Geometry check sheet. Reference: drawing and pictorial views, mm from the part's lowest x, y, z. A direction names the side the tool comes from. Coordinates: 2 decimals unless noted, no trailing zeros. Order: outer loops, then holes, each group sorted by start corner. A loop starts at its lowest first (then second) coordinate and runs counter-clockwise, first axis right, second up. Notation, with made-up numbers: (55.5, 19) -> (97.5, 19) arc R26 ccw to (97.5, 33) -> close; hole circle Ø6 at (75.5, 74.25). An arc over 180 degrees is marked (long way). Use CSV: the item, a comma, the result in double quotes. Start each with the question number.
1) Go/stop test with flat-tipped pins: pin 1 (6 mm diameter, centred on y = 17, z = 14, fed in from +X) (1 decimal); pin 2 (2 mm diameter, centred on y = 9, z = 3.5, fed in from +X); pin 3 (5 mm diameter, centred on x = 4.5, z = 12, fed in from +Y); pin 4 (1.8 mm diameter, centred on x = 21.08, y = 7.86, fed in from -Z). Record where each tip stops, or that it passes through.
2) Tool access check on the marked faces 1 and 2. Record the directions out of +Z, -Z, +X, -X, +Y, -Y that give a thin tool (end or side, any length) a straight path to the whole face; none if there is none.
3) Scan lines: line 1 along Y through (x, z) = (12.7, 2.1); line 2 along Z through (x, y) = (18.5, 3.5); line 3 along Y through (x, z) = (3.25, 2.5) (1 decimal). Record each from-to range of solid material in increasing order.
4) Sectioned sample at B-B on x = 12.7. Give the number of separate pieces and of enclosed holes in the cut face.
5) Sectioned sample at A-A on y = 12.7. Record the boundary of the cut face in (x, z).
6) Sectioned sample at C-C on z = 7. Record the boundary of the cut face in (x, y).
7) Sectioned sample at D-D on y = 15.25. Record the boundary of the cut face in (x, z) (1 decimal), then the cut area to 3 significant figures.
8) Release check for a two-part mould opening along Y. For the marked faces 3, 4 and 5 record: released by +Y, released by -Y, zero draft, split by the parting line, or undercut.
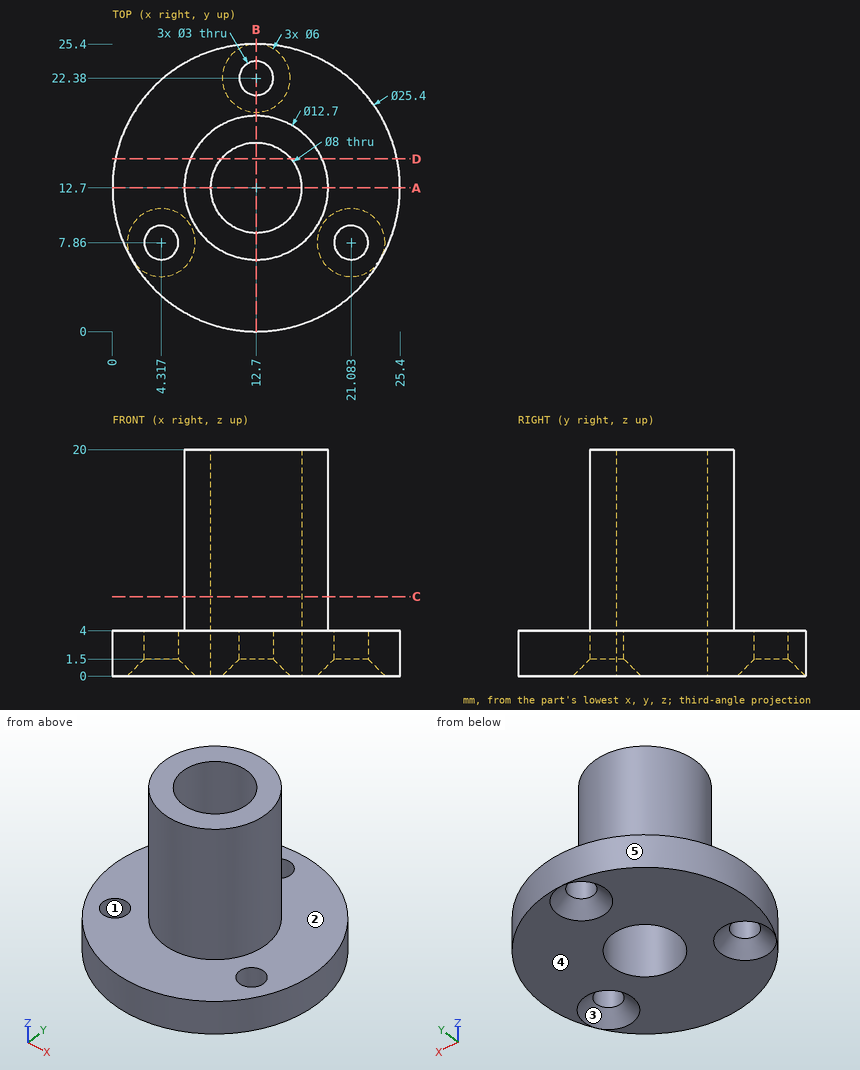
Answers follow:
1,pin 1,"stops at x = 18.9"
1,pin 2,"stops at x = 25.11"
1,pin 3,"stops at y = 15.5"
1,pin 4,"passes through"
2,face 1,"+Z, -Z"
2,face 2,"+Z"
3,line 1,"y = 0 to 8.7, 16.7 to 20.88, 23.88 to 25.4"
3,line 2,"z = 0 to 4"
3,line 3,"y = 4.2 to 6.8, 8.9 to 21.2"
4,separate pieces,"3"
4,enclosed holes,"0"
5,outline,"(0, 0) -> (8.7, 0) -> (8.7, 20) -> (6.35, 20) -> (6.35, 4) -> (0, 4) -> close; (16.7, 0) -> (25.4, 0) -> (25.4, 4) -> (19.05, 4) -> (19.05, 20) -> (16.7, 20) -> close"
6,outline,"circle Ø12.7 at (12.7, 12.7); hole circle Ø8 at (12.7, 12.7)"
7,outline,"(0.3, 0) -> (9.6, 0) -> (9.6, 20) -> (6.9, 20) -> (6.9, 4) -> (0.3, 4) -> close; (15.8, 0) -> (25.1, 0) -> (25.1, 4) -> (18.5, 4) -> (18.5, 20) -> (15.8, 20) -> close"
7,area,"162 mm²"
8,face 3,"undercut"
8,face 4,"zero draft"
8,face 5,"split by the parting line"
